Could you check a few things on this drawing? It's one solid part, dimensions in mm from its lowest x, y, z. A direction names the side the tool comes from. Give positions to 0.01 mm unless a question says otherwise; leave off trailing zeros. Write each loop counter-clockwise with the first axis right and the second up, starting at its lowest first coordinate (ties: lowest second). Pieces come first, ordered by that corner, then holes.
1. If I drill on probe 1 along Z at (x, y) = (12, 8); probe 2 along Y at (x, z) = (16, 1.25), over which ranges is the centre line in solid material (lowest first)?
2. Suppose I cut it at A-A (x = 16). Please give me the cut outline in (y, z), and give its area (3 significant figures).
3. Suppose I cut it at C-C (y = 24). Please give me the cut outline in (x, z), and give its area (3 significant figures).
4. Thinking about a two-plate mould opening in X: for the marked faces 4, 5, 6 and 7, which applies, pulls with the +X half, pulls with the -X half, needs draft (parallel to the pull), parting line crosses it, or undercut?
5. On a 3-axis mill with a long thin cutter (end or side, diameter ignored), from which of +Z, -Z, +X, -X, +Y, -Y can I reach the whole of each face in a straight line? I mean the marked faces 1, 2 and 3. Say none if no direction works.
6. Suppose I cut it at B-B (z = 15). Please give me the cut outline in (x, y).
7. Suppose I cut it at D-D (x = 9). Please give me the cut outline in (y, z), and give its area (3 significant figures).
8. I'm going to push flat-ended pins straight in: pin 1 (1.5 mm diameter, centred on x = 16.5, y = 3.5, fed in from +Z); pin 2 (0.9 mm diameter, centred on x = 3, z = 15, fed in from +Y); pin 3 (4 mm diameter, centred on y = 4, z = 21.5, fed in from +X). Where does each tip first touch, or does it pass through?
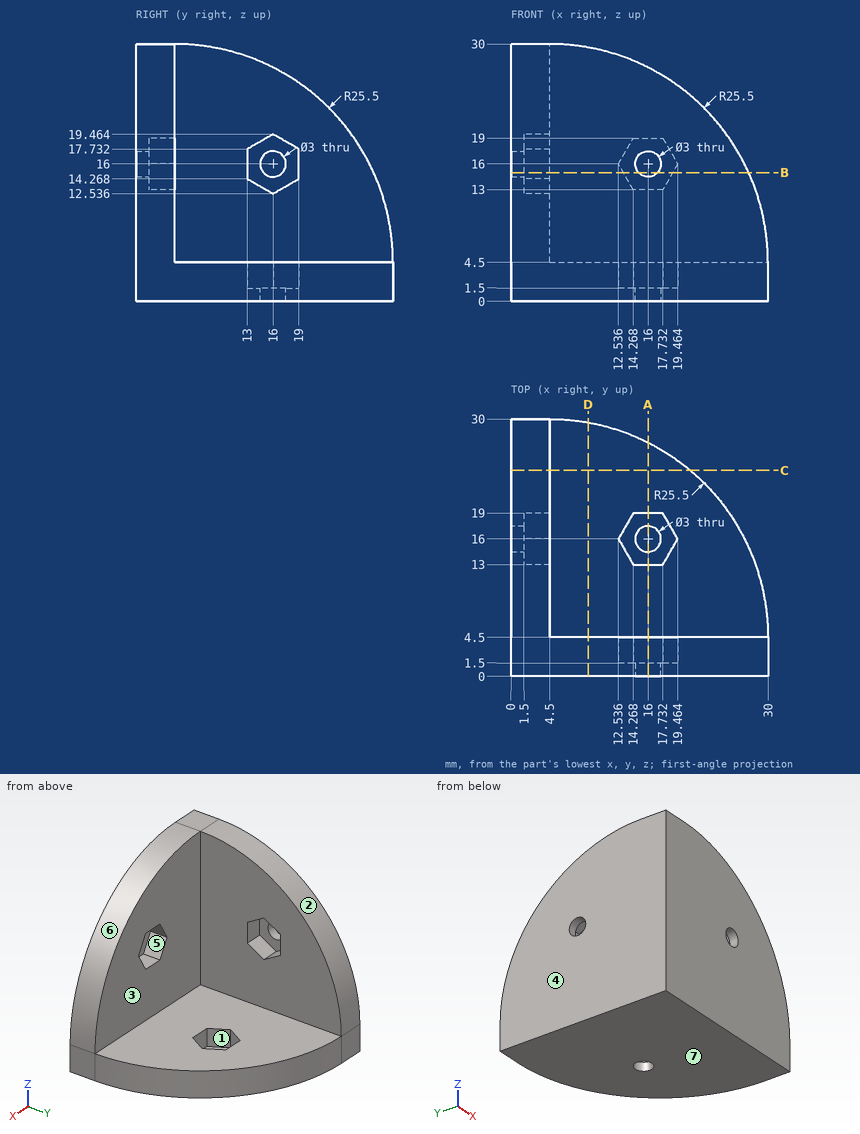
Checks:
1. probe 1: z = 0 to 4.5
1. probe 2: y = 0 to 14.5, 17.5 to 27.26
2. outline: (0, 0) - (14.5, 0) - (14.5, 1.5) - (13, 1.5) - (13, 4.5) - (4.5, 4.5) - (4.5, 13) - (1.5, 13) - (1.5, 14.5) - (0, 14.5) - close; (0, 17.5) - (1.5, 17.5) - (1.5, 19) - (4.5, 19) - (4.5, 27.26) - (0, 27.26) - close; (17.5, 0) - (27.26, 0) - (27.26, 4.5) - (19, 4.5) - (19, 1.5) - (17.5, 1.5) - close
2. area: 180 mm2
3. outline: (0, 0) - (20.93, 0) - (20.93, 4.5) - (4.5, 4.5) - (4.5, 20.93) - (0, 20.93) - close
3. area: 168 mm2
4. face 4: pulls with the -X half
4. face 5: undercut
4. face 6: pulls with the +X half
4. face 7: needs draft
5. face 1: +Z
5. face 2: +Z, +X, -X, +Y
5. face 3: +Z, +X, +Y
6. outline: (0, 0) - (14.88, 0) - (14.88, 1.5) - (13.11, 1.5) - (13.11, 4.5) - (4.5, 4.5) - (4.5, 13) - (1.5, 13) - (1.5, 14.88) - (0, 14.88) - close; (0, 17.12) - (1.5, 17.12) - (1.5, 19) - (4.5, 19) - (4.5, 27.74) - (0, 27.74) - close; (17.12, 0) - (27.74, 0) - (27.74, 4.5) - (18.89, 4.5) - (18.89, 1.5) - (17.12, 1.5) - close
7. outline: (0, 0) - (29.6, 0) - (29.6, 4.5) - (4.5, 4.5) - (4.5, 29.6) - (0, 29.6) - close
7. area: 246 mm2
8. pin 1: stops at z = 27.38
8. pin 2: stops at y = 27.94
8. pin 3: stops at x = 25.12
